Part model, mm, in its own coordinate system. A direction names the side the tool comes from. Coordinates: 2 decimals unless noted, no trailing zeros. Loops run counter-clockwise (first coordinate to the right, second up) from the corner with the lowest first, then second, coordinate; pieces in that order, holes last. Notation, with made-up numbers: (-28.5, 23.25) - (19.5, 23.25) arc R16 cw to (19.5, 33.25) - close; hole circle Ø5 at (-16.75, -30.75). An arc over 180 degrees is marked (long way). Answer as CSV lines item,"result".
from build123d import *

# Parameters (mm, degrees)
SKETCH1_R           = 15
BOSS_EXTRUDE1_DEPTH = 20
SKETCH2_R           = 8
CUT_EXTRUDE1_DEPTH  = 5
SKETCH4_W           = 65
SKETCH4_H           = 65
BOSS_EXTRUDE2_DEPTH = 5
SKETCH3_R           = 6
CUT_EXTRUDE2_DEPTH  = 51.124844139
SKETCH5_R           = 1.75
CUT_EXTRUDE3_DEPTH  = 49.347699015
SKETCH6_R           = 1.75
CUT_EXTRUDE4_DEPTH  = 51.124844139


with BuildPart() as part:
    # Sketch1 → Boss-Extrude1 (new body)
    with BuildSketch(Plane.XY):
        Circle(SKETCH1_R)
    extrude(amount=-BOSS_EXTRUDE1_DEPTH)

    # Sketch2 → Cut-Extrude1 (cut)
    with BuildSketch(Plane(origin=(0, 0, -20), x_dir=(-1, 0, 0), z_dir=(0, 0, -1))):
        Circle(SKETCH2_R)
    extrude(amount=-CUT_EXTRUDE1_DEPTH, mode=Mode.SUBTRACT)

    # Sketch4 → Boss-Extrude2 (add)
    with BuildSketch(Plane.XY):
        Rectangle(SKETCH4_W, SKETCH4_H)
    extrude(amount=-BOSS_EXTRUDE2_DEPTH)

    # Sketch3 → Cut-Extrude2 (cut, through all)
    with BuildSketch(Plane.XY):
        Circle(SKETCH3_R)
    extrude(amount=-CUT_EXTRUDE2_DEPTH, mode=Mode.SUBTRACT)

    # Sketch5 → Cut-Extrude3 (cut, through all)
    with BuildSketch(Plane(origin=(0, 0, -5), x_dir=(-1, 0, 0), z_dir=(0, 0, -1))):
        with Locations((-28.25, 29)):
            Circle(SKETCH5_R)
        with Locations(Location((28.25, 29, 0), (0, 0, 180))):
            Circle(SKETCH5_R)
        with Locations((28.25, -29)):
            Circle(SKETCH5_R)
        with Locations(Location((-28.25, -29, 0), (0, 0, 180))):
            Circle(SKETCH5_R)
    extrude(amount=-CUT_EXTRUDE3_DEPTH, mode=Mode.SUBTRACT)

    # Sketch6 → Cut-Extrude4 (cut, through all)
    with BuildSketch(Plane.XY):
        with Locations((0, 19)):
            Circle(SKETCH6_R)
        with Locations((0, -19)):
            Circle(SKETCH6_R)
    extrude(amount=-CUT_EXTRUDE4_DEPTH, mode=Mode.SUBTRACT)


solid = part.part
Q1. Saw through at C-C (z = -2.75). Give the cut face in (x, y).
Results:
outline,"(-32.5, -32.5) - (32.5, -32.5) - (32.5, 32.5) - (-32.5, 32.5) - close; hole circle Ø3.5 at (-28.25, -29); hole circle Ø3.5 at (-28.25, 29); hole circle Ø12 at (0, 0); hole circle Ø3.5 at (0, -19); hole circle Ø3.5 at (0, 19); hole circle Ø3.5 at (28.25, -29); hole circle Ø3.5 at (28.25, 29)"
Q2. Wall check: L1, parallel to Y at x = 28.25, z = -2.85; L2, parallel to Z at x = 16.5, y = 14; L3, parallel to X at y = 1.5, z = -8.25. Give the ranges that are in metal, low to high.
Results:
L1,"y = -32.5 to -30.75, -27.25 to 27.25, 30.75 to 32.5"
L2,"z = -5 to 0"
L3,"x = -14.92 to -5.81, 5.81 to 14.92"
Q3. Saw through at A-A (x = 28.25). Give the cut face in (y, z), then the cut area to 3 significant figures.
Results:
outline,"(-32.5, -5) - (-30.75, -5) - (-30.75, 0) - (-32.5, 0) - close; (-27.25, -5) - (27.25, -5) - (27.25, 0) - (-27.25, 0) - close; (30.75, -5) - (32.5, -5) - (32.5, 0) - (30.75, 0) - close"
area,"290 mm^2"
Q4. Saw through at D-D (x = 0). Give the cut face in (y, z).
Results:
outline,"(-32.5, -5) - (-20.75, -5) - (-20.75, 0) - (-32.5, 0) - close; (-17.25, -5) - (-15, -5) - (-15, -20) - (-8, -20) - (-8, -15) - (-6, -15) - (-6, 0) - (-17.25, 0) - close; (6, -15) - (8, -15) - (8, -20) - (15, -20) - (15, -5) - (17.25, -5) - (17.25, 0) - (6, 0) - close; (20.75, -5) - (32.5, -5) - (32.5, 0) - (20.75, 0) - close"
Q5. Two-plate mould, pull along X, no slides. Class faces 3 (the face through (32.5, 0, -2)), 4 (the face through (-8, 15, -5)), 5 (the face through (-30, 29, -3)): released by +X, released by -X, zero draft, split by the parting line, or undercut.
Results:
face 3,"released by +X"
face 4,"zero draft"
face 5,"undercut"
Q6. Saw through at B-B (y = -29). Give the cut face in (x, z), then the cut area to 3 significant figures.
Results:
outline,"(-32.5, -5) - (-30, -5) - (-30, 0) - (-32.5, 0) - close; (-26.5, -5) - (26.5, -5) - (26.5, 0) - (-26.5, 0) - close; (30, -5) - (32.5, -5) - (32.5, 0) - (30, 0) - close"
area,"290 mm^2"
Q7. Which spindle directions (+Z, -Z, +X, -X, +Y, -Y) get a long thin tool onto all of the face, cutting with end or side? Do faces 1 (the face through (-8, 0, 0)), 2 (the face through (1.73, -7.81, -17.54)). Say none if no direction does.
Results:
face 1,"+Z, +X, -X, +Y, -Y"
face 2,"-Z"
Q8. Flat gauge pins, fed straight in: pin 1 (15.5 mm diameter, centred on x = 0, y = 0, fed in from -Z); pin 2 (5 mm diameter, centred on x = 24, y = -12.5, fed in from -Z); pin 3 (2 mm diameter, centred on x = 3.5, z = -12.5, fed in from -Y). Where does each tip first touch, or does it go through?
Results:
pin 1,"stops at z = -15"
pin 2,"stops at z = -5"
pin 3,"stops at y = -14.79"
